Check sheet for the modelled part. Datum: model origin and axes. Units: mm. Round coordinates to 2 decimals unless told otherwise and drop trailing zeros. Write each loop counter-clockwise with the first axis right and the second up, starting at its lowest first coordinate (ties: lowest second). Pieces come first, ordered by that corner, then holes. Notation, with made-up numbers: (32, 62.25) -> (65, 62.25) arc R28 ccw to (65, 99.25) -> close; hole circle Ø5 at (67.5, -24). An arc over 180 degrees is marked (long way). One line per item, written item: value.
from build123d import *

# Parameters (mm, degrees)
SKIZZE1_R                       = 30.405
SKIZZE1_R_2                     = 28.405
AUFSATZ_LINEAR_AUSTRAGEN1_DEPTH = 10
SKIZZE2_R                       = 30.405
AUFSATZ_LINEAR_AUSTRAGEN2_DEPTH = 1
AUFSATZ_LINEAR_START            = 10
AUFSATZ_LINEAR_AUSTRAGEN3_DEPTH = 10
SKIZZE5_R                       = 1.5
SCHNITT_LINEAR_AUSTRAGEN2_DEPTH = 10
SKIZZE6_W                       = 7.2
SKIZZE6_H                       = 10
SCHNITT_LINEAR_AUSTRAGEN3_DEPTH = 10
KREISMUSTER1_COUNT              = 2
KREISMUSTER1_ANGLE              = 90


with BuildPart() as part:
    # Skizze1 → Aufsatz-Linear austragen1 (new body)
    with BuildSketch(Plane(origin=(0, 0, 0), x_dir=(1, 0, 0), z_dir=(0, 1, 0))):
        with Locations(Location((0, 0, 0), (0, 0, 270))):
            Circle(SKIZZE1_R)
        with Locations(Location((0, 0, 0), (0, 0, 270))):
            Circle(SKIZZE1_R_2, mode=Mode.SUBTRACT)
    extrude(amount=AUFSATZ_LINEAR_AUSTRAGEN1_DEPTH)

    # Skizze2 → Aufsatz-Linear austragen2 (add)
    with BuildSketch(Plane(origin=(0, 10, 0), x_dir=(1, 0, 0), z_dir=(0, 1, 0))):
        with Locations(Location((0, 0, 0), (0, 0, 270))):
            Circle(SKIZZE2_R)
    extrude(amount=AUFSATZ_LINEAR_AUSTRAGEN2_DEPTH)

    # Skizze4 → Aufsatz-Linear austragen3 (add)
    with BuildSketch(Plane.XZ.offset(-10).offset(AUFSATZ_LINEAR_START)):
        with BuildLine():
            ThreePointArc((-28.126789531, -3.965820935), (-23.605, 0), (-28.126789531, 3.965820935))
            ThreePointArc((-28.126789531, 3.965820935), (-28.405, 0), (-28.126789531, -3.965820935))
        make_face()
        with BuildLine():
            ThreePointArc((28.405, 0), (28.33536202, 1.987783738), (28.126789531, 3.965820935))
            ThreePointArc((28.126789531, 3.965820935), (23.605, 0), (28.126789531, -3.965820935))
            ThreePointArc((28.126789531, -3.965820935), (28.33536202, -1.987783738), (28.405, 0))
        make_face()
    aufsatz_linear_austragen3 = extrude(amount=-AUFSATZ_LINEAR_AUSTRAGEN3_DEPTH)

    # Skizze5 → Schnitt-Linear austragen2 (cut)
    with BuildSketch(Plane.XZ):
        with Locations(Location((-27.605, 0, 0), (0, 0, 270))):
            Circle(SKIZZE5_R)
        with BuildLine():
            ThreePointArc((29.105, 0), (27.605, 1.5), (26.105, 0))
            Line((26.105, 0), (29.105, 0))
        make_face()
        with BuildLine():
            Line((29.105, 0), (26.105, 0))
            ThreePointArc((26.105, 0), (27.605, -1.5), (29.105, 0))
        make_face()
    schnitt_linear_austragen2 = extrude(amount=-SCHNITT_LINEAR_AUSTRAGEN2_DEPTH, mode=Mode.SUBTRACT)

    # Skizze6 → Schnitt-Linear austragen3 (cut)
    with BuildSketch(Plane(origin=(0, 11, 0), x_dir=(1, 0, 0), z_dir=(0, 1, 0))):
        with Locations((-6.308057451, -13.288570201)):
            Rectangle(SKIZZE6_W, SKIZZE6_H)
    extrude(amount=-SCHNITT_LINEAR_AUSTRAGEN3_DEPTH, mode=Mode.SUBTRACT)

    # Kreismuster1: Aufsatz-Linear austragen3, Schnitt-Linear austragen2 ×2 about axis
    kreismuster1_axis = Axis((0, 0, 0), (0, 1, 0))
    add([aufsatz_linear_austragen3.rotate(kreismuster1_axis, i * KREISMUSTER1_ANGLE / (KREISMUSTER1_COUNT - 1)) for i in range(1, KREISMUSTER1_COUNT)])
    add([schnitt_linear_austragen2.rotate(kreismuster1_axis, i * KREISMUSTER1_ANGLE / (KREISMUSTER1_COUNT - 1)) for i in range(1, KREISMUSTER1_COUNT)], mode=Mode.SUBTRACT)


solid = part.part
Item 1: Sectioned sample at D-D (x = -6.5). Enter the section's corners in (y, z).
Result set:
outline: (0, -29.7) -> (11, -29.7) -> (11, 8.29) -> (10, 8.29) -> (10, -27.65) -> (0, -27.65) -> close; (0, 27.65) -> (10, 27.65) -> (10, 18.29) -> (11, 18.29) -> (11, 29.7) -> (0, 29.7) -> close
Item 2: Release check for a two-part mould opening along Z. For faces 1 (the cylindrical face through (19.9, 4.93, 20.27)), 2 (the cylindrical face through (-18.5, 5.42, -24.13)), 3 (the flat face through (0, 11, 0)) record: pulls with the +Z half, pulls with the -Z half, needs draft (parallel to the pull), parting line crosses it, or undercut.
Result set:
face 1: undercut
face 2: parting line crosses it
face 3: needs draft
Item 3: Material ranges on line 1 along Z through (x, y) = (0.5, 6); line 2 along Z through (x, y) = (24.5, 9.75); line 3 along Y through (x, z) = (15, 0), recorded low to high.
Result set:
line 1: -30.4 to -29.02, -26.19 to -23.64, 23.64 to 26.19, 29.02 to 30.4
line 2: -18.01 to -14.37, -2.52 to 2.52, 14.37 to 18.01
line 3: 10 to 11
Item 4: Depth check by flat-ended pin: pin 1 (6 mm diameter, centred on y = 10, z = -14.5, fed in from +X); pin 2 (1.5 mm diameter, centred on x = 0, z = 27, fed in from -Y); pin 3 (4 mm diameter, centred on y = 2, z = 6.5, fed in from +X). Enter the tip coordinate at first touch or a pass-through.
Result set:
pin 1: x = 28.15
pin 2: y = 10
pin 3: x = 30.07
Item 5: Sectioned sample at A-A (z = 0). Enter the section's corners in (x, y) (3 decimals).
Result set:
outline: (-30.405, 0) -> (-29.105, 0) -> (-29.105, 10) -> (-26.105, 10) -> (-26.105, 0) -> (-23.605, 0) -> (-23.605, 10) -> (23.605, 10) -> (23.605, 0) -> (26.105, 0) -> (26.105, 10) -> (29.105, 10) -> (29.105, 0) -> (30.405, 0) -> (30.405, 11) -> (-30.405, 11) -> close
Item 6: Sectioned sample at B-B (x = 0). Enter the section's corners in (y, z) (3 decimals).
Result set:
outline: (0, -30.405) -> (11, -30.405) -> (11, 30.405) -> (0, 30.405) -> (0, 29.105) -> (10, 29.105) -> (10, 26.105) -> (0, 26.105) -> (0, 23.605) -> (10, 23.605) -> (10, -23.605) -> (0, -23.605) -> (0, -26.105) -> (10, -26.105) -> (10, -29.105) -> (0, -29.105) -> close
Item 7: Sectioned sample at C-C (y = 4.25). Enter the section's corners in (x, z) (3 decimals).
Result set:
outline: circle Ø60.81 at (0, 0); hole circle Ø3 at (-27.605, 0); hole (-28.127, -3.966) arc R28.405 ccw to (-3.966, -28.127) arc R4 cw (long way) to (3.966, -28.127) arc R28.405 ccw to (28.127, -3.966) arc R4 cw (long way) to (28.127, 3.966) arc R28.405 ccw to (3.966, 28.127) arc R4 cw (long way) to (-3.966, 28.127) arc R28.405 ccw to (-28.127, 3.966) arc R4 cw (long way) to start; hole circle Ø3 at (0, -27.605); hole circle Ø3 at (0, 27.605); hole circle Ø3 at (27.605, 0)
